Source: CAD feature listing. Evaluate the final solid. Frame: model axes, mm. A direction names the side the tool comes from. Round coordinates to 2 decimals unless told otherwise and drop trailing zeros. Loops run counter-clockwise (first coordinate to the right, second up) from the corner with the lowest first, then second, coordinate; pieces in that order, holes last.
Item 1: Section query B-B on y = -33. Return loops of the section in (x, z), then the cut area to 3 significant figures.
Item 2: First-contact query: P1, Ø12, axis at x = 223, y = -23, coming from the -Z side; P2, Ø15.5, axis at x = 638, z = 3.5, coming from the +Y side; P3, Ø18, axis at x = -90, z = -25, coming from the -Y side; P4, Ø4, axis at y = -10, z = 52, coming from the -X side. Flat tips, straight axial feed; report the tip coordinate or a pass-through.
Item 3: Section query A-A on x = -180. Return loops of the section in (y, z), then the cut area to 3 significant figures.
Item 4: Section query C-C on x = 209.5. Return loops of the section in (y, z), then the cut area to 3 significant figures.
Item 5: Section query D-D on x = 949. Return loops of the section in (y, z), then the cut area to 3 significant figures.
Item 6: Ray query, L1, parallel to X at y = 6, z = -25; L2, parallel to Y at x = 154, z = -13; L3, parallel to X at y = 12.5, z = -23. Return the intervals inside material, ascending.
Item 7: Access query for faces 1 (the flat face through (760, 0, 0)), 2 (the flat face through (40, -25, 1)), 3 (the flat face through (-87, 35, -1)). Directions: +Z, -Z, +X, -X, +Y, -Y. A direction counts if a zero-diameter tool reaches every point of the face in a straight line with its end or side. Return the directions, or none.
Item 8: Pull-direction query (Z, two-part tool) for faces 4 (the flat face through (-87, -45, -1)), 5 (the flat face through (760, -5, 8)); classes: released by +Z, released by -Z, zero draft, split by the parting line, or undercut.
```python
from build123d import *

# Parameters (mm, degrees)
BOSS_EXTRUDE1_DEPTH      = 1500
FILLET1_R                = 40
FILLET2_R                = 40
FILLET3_R                = 5
FILLET4_R                = 5
CUT_EXTRUDE1_DEPTH       = 1502.3316039943886
CUT_EXTRUDE1_DEPTH_BACK  = 1502.3316039943886
FILLET5_R                = 25
BOSS_EXTRUDE2_DEPTH      = 35
BOSS_EXTRUDE2_DEPTH_BACK = 45
SKETCH3_R                = 15.000000000000025
SKETCH3_R_2              = 14.999999999999998


with BuildPart() as part:
    # Sketch1 → Boss-Extrude1 (new body)
    with BuildSketch(Plane(origin=(0, 0, 0), x_dir=(0, 0, -1), z_dir=(1, 0, 0))):
        Polygon((0, 0), (40, 0), (61.94779998780638, -18.416390874921095), (58.733861939373675, -22.246613090515982), (38.18014882866898, -5), (0, -5), (-38.18014882866898, -5), (-58.733861939373675, -22.246613090515982), (-61.94779998780638, -18.416390874921095), (-40, 0), align=None)
    extrude(amount=BOSS_EXTRUDE1_DEPTH)

    # Fillet1
    fillet1_edges = [part.edges().sort_by_distance(p)[0] for p in [
        (750, -5, -38.18014882866898),
        (750, 0, 40),
    ]]
    fillet(fillet1_edges, radius=FILLET1_R)

    # Fillet2
    fillet2_edges = [part.edges().sort_by_distance(p)[0] for p in [
        (750, 0, -40),
    ]]
    fillet(fillet2_edges, radius=FILLET2_R)

    # Fillet3
    # the kernel refuses this fillet: 5 mm, written as the material it takes off along each edge
    with BuildSketch(Plane(origin=(0, -8.840835335933875, -69.98264510888814), x_dir=(0, 0.6427876096865403, 0.7660444431189772), z_dir=(0, -0.7660444431189772, 0.6427876096865403))) as fillet3_piece_1:
        with BuildLine():
            CenterArc((FILLET3_R, -FILLET3_R), FILLET3_R, 90, 90)
            Line((-2.28e-15, -FILLET3_R), (0, 0))
            Line((0, 0), (FILLET3_R, 0))
        make_face()
    extrude(amount=30.000000000000007, mode=Mode.SUBTRACT)
    with BuildSketch(Plane(origin=(-12.500000000000002, -18.4163908749211, -61.94779998780638), x_dir=(0, 0.6427876096865406, 0.7660444431189771), z_dir=(1, 0, 0))) as fillet3_piece_2:
        with BuildLine():
            CenterArc((FILLET3_R, FILLET3_R), FILLET3_R, 180, 90)
            Line((1.03e-15, FILLET3_R), (0, 0))
            Line((0, 0), (FILLET3_R, 2.8e-16))
        make_face()
    extrude(amount=1525, mode=Mode.SUBTRACT)
    with BuildSketch(Plane(origin=(-12.500000000000002, -22.246613090515982, -58.733861939373675), x_dir=(0, 0.7660444431189772, -0.6427876096865403), z_dir=(1, 0, 0))) as fillet3_piece_3:
        with BuildLine():
            CenterArc((FILLET3_R, FILLET3_R), FILLET3_R, 180, 90)
            Line((1.1e-16, FILLET3_R), (0, 0))
            Line((0, 0), (FILLET3_R, -6e-17))
        make_face()
    extrude(amount=1525, mode=Mode.SUBTRACT)
    with BuildSketch(Plane(origin=(1500, -8.840835335933875, -69.98264510888814), x_dir=(0, 0.6427876096865403, 0.7660444431189772), z_dir=(0, -0.7660444431189772, 0.6427876096865403))) as fillet3_piece_4:
        with BuildLine():
            CenterArc((FILLET3_R, FILLET3_R), FILLET3_R, 180, 90)
            Line((-2.28e-15, FILLET3_R), (0, 0))
            Line((0, 0), (FILLET3_R, 0))
        make_face()
    extrude(amount=30.000000000000007, mode=Mode.SUBTRACT)

    # Fillet4
    # the kernel refuses this fillet: 5 mm, written as the material it takes off along each edge
    with BuildSketch(Plane(origin=(0, -31.822168629503203, 50.69901681829192), x_dir=(0, 0.6427876096865403, -0.7660444431189772), z_dir=(0, 0.7660444431189772, 0.6427876096865403))) as fillet4_piece_1:
        with BuildLine():
            CenterArc((FILLET4_R, -FILLET4_R), FILLET4_R, 90, 90)
            Line((0, -FILLET4_R), (0, 0))
            Line((0, 0), (FILLET4_R, 0))
        make_face()
    extrude(amount=30.000000000000007, mode=Mode.SUBTRACT)
    with BuildSketch(Plane(origin=(-12.500000000000007, -22.246613090515982, 58.733861939373675), x_dir=(0, 0.7660444431189776, 0.6427876096865399), z_dir=(1, 0, 0))) as fillet4_piece_2:
        with BuildLine():
            CenterArc((FILLET4_R, -FILLET4_R), FILLET4_R, 90.00000000000004, 90)
            Line((5.38e-15, -FILLET4_R), (0, 0))
            Line((0, 0), (FILLET4_R, 2.4e-16))
        make_face()
    extrude(amount=1525, mode=Mode.SUBTRACT)
    with BuildSketch(Plane(origin=(-12.500000000000002, -18.416390874921095, 61.94779998780638), x_dir=(0, 0.6427876096865403, -0.7660444431189772), z_dir=(1, 0, 0))) as fillet4_piece_3:
        with BuildLine():
            CenterArc((FILLET4_R, -FILLET4_R), FILLET4_R, 90, 89.99999999999997)
            Line((2.28e-15, -FILLET4_R), (0, 0))
            Line((0, 0), (FILLET4_R, 1.1e-16))
        make_face()
    extrude(amount=1525, mode=Mode.SUBTRACT)
    with BuildSketch(Plane(origin=(1500, -31.822168629503203, 50.69901681829192), x_dir=(0, 0.6427876096865403, -0.7660444431189772), z_dir=(0, 0.7660444431189772, 0.6427876096865403))) as fillet4_piece_4:
        with BuildLine():
            CenterArc((FILLET4_R, FILLET4_R), FILLET4_R, 180, 90)
            Line((0, FILLET4_R), (0, 0))
            Line((0, 0), (FILLET4_R, 0))
        make_face()
    extrude(amount=30.000000000000007, mode=Mode.SUBTRACT)

    # Sketch2 → Cut-Extrude1 (cut, two sides: drawn at the far end of the back side and taken through both)
    with BuildSketch(Plane(origin=(0, 0, 0), x_dir=(1, 0, 0), z_dir=(0, 1, 0)).offset(-CUT_EXTRUDE1_DEPTH_BACK)):
        Polygon((1500, -59.90363972377879), (1500, -25.441190629351873), (101.5742667563142, -59.90363972377879), align=None)
        Polygon((1500, 59.90363972377879), (1500, 25.441190629351873), (101.57426675631426, 59.90363972377879), align=None)
    extrude(amount=CUT_EXTRUDE1_DEPTH + CUT_EXTRUDE1_DEPTH_BACK, mode=Mode.SUBTRACT)

    # Fillet5
    fillet5_edges = [part.edges().sort_by_distance(p)[0] for p in [
        (1500, -2.5207098367195613, -25.441190629351873),
        (1500, -2.5, 25.441190629351873),
    ]]
    fillet(fillet5_edges, radius=FILLET5_R)

    # Sketch3 → Boss-Extrude2 (add, two sides: drawn at the far end of the back side and taken through both)
    with BuildSketch(Plane(origin=(0, 0, 0), x_dir=(1, 0, 0), z_dir=(0, 1, 0)).offset(-BOSS_EXTRUDE2_DEPTH_BACK)):
        Polygon((39.99999999999999, 45.00000000000001), (-210, 44.99999999999998), (-210, -45.00000000000002), (40.00000000000001, -44.99999999999998), align=None)
        with Locations(Location((-180, -1.78e-15, 0), (0, 0, 270))):
            Circle(SKETCH3_R, mode=Mode.SUBTRACT)
        with Locations(Location((-90, 25, 0), (0, 0, 270))):
            Circle(SKETCH3_R_2, mode=Mode.SUBTRACT)
        with Locations(Location((-90, -25, 0), (0, 0, 270))):
            Circle(SKETCH3_R_2, mode=Mode.SUBTRACT)
    extrude(amount=BOSS_EXTRUDE2_DEPTH + BOSS_EXTRUDE2_DEPTH_BACK)


solid = part.part
```
Data:
1. outline: (-210, -45) - (40, -45) - (40, 45) - (-210, 45) - close; hole circle Ø30 at (-180, 0); hole circle Ø30 at (-90, -25); hole circle Ø30 at (-90, 25)
1. area: 20,400 mm2
2. P1: stops at z = -57.04
2. P2: stops at y = 0
2. P3: passes through
2. P4: stops at x = 0
3. outline: (-45, -45) - (35, -45) - (35, -15) - (-45, -15) - close; (-45, 15) - (35, 15) - (35, 45) - (-45, 45) - close
3. area: 4,800 mm2
4. outline: (-20.13, -57.24) - (-14.47, -57.24) - (-9.36, -51.15) arc R40 ccw to (0, -25.44) - (0, 25.44) arc R40 ccw to (-9.36, 51.15) - (-14.47, 57.24) - (-20.13, 57.24) arc R5 ccw to (-19.03, 54.9) - (-5, 38.18) - (-5, -23.62) arc R40 cw to (-14.36, -49.33) - (-19.03, -54.9) arc R5 ccw to start
4. area: 603 mm2
5. outline: (-8.08, -39.02) - (-2.38, -39.02) arc R40 ccw to (0, -25.44) - (0, 25.44) arc R40 ccw to (-2.38, 39.02) - (-5.7, 39.02) - (-5, 38.18) - (-5, -23.62) arc R40 cw to start
5. area: 385 mm2
6. L1: x = -210 to -105, -75 to 40
6. L2: y = -5 to 0
6. L3: x = -210 to -104.87, -75.13 to 40
7. face 1: +Z, -Z, +X, +Y
7. face 2: +X, -Y
7. face 3: +Z, -Z, +X, -X, +Y
8. face 4: zero draft
8. face 5: undercut
